Check sheet for the drawn part. Datum: minimum x, y, z corner. Units: mm. Round coordinates to 2 decimals unless told otherwise and drop trailing zeros. Write each loop counter-clockwise with the first axis right and the second up, starting at its lowest first coordinate (ties: lowest second). Pieces come first, ordered by that corner, then holes. Notation, with made-up numbers: (29, 5.25) - (73, 5.25) arc R16 cw to (73, 10.25) - close; hole circle Ø3 at (67, 68.5). An arc over 180 degrees is marked (long way). Write each question's results on one line, items separated by ' | '.
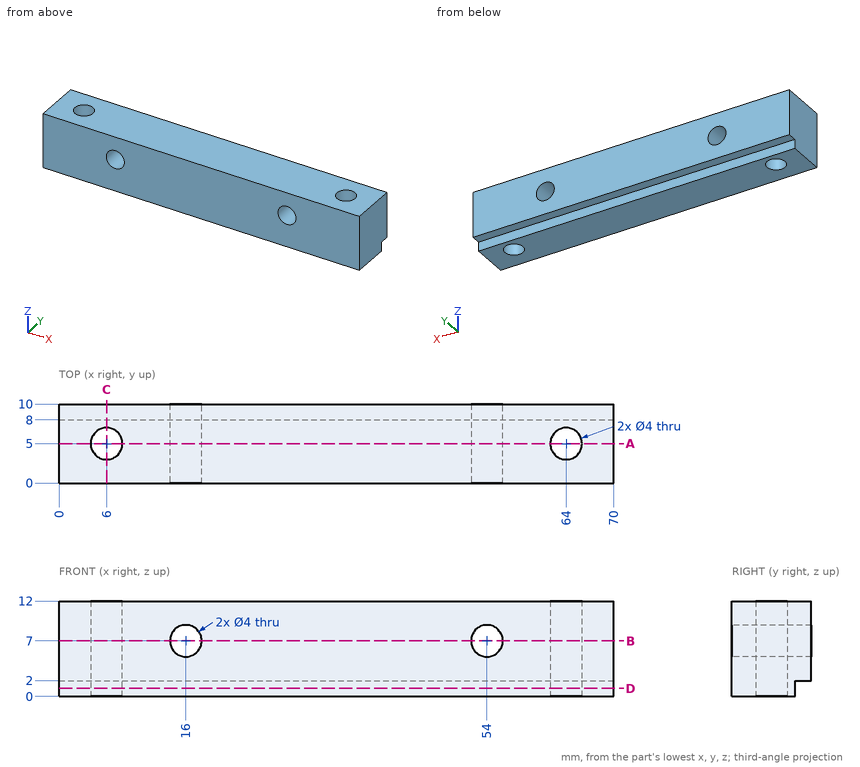
(1) Section check D-D (z = 1). Record the cut outline in (x, y), plus the area to 3 significant figures.
Answer:
outline: (0, 0) - (70, 0) - (70, 8) - (0, 8) - close; hole circle Ø4 at (6, 5); hole circle Ø4 at (64, 5) | area: 535 mm2
(2) Section check B-B (z = 7). Record the cut outline in (x, y), plus the area to 3 significant figures.
Answer:
outline: (0, 0) - (14, 0) - (14, 10) - (0, 10) - close; (18, 0) - (52, 0) - (52, 10) - (18, 10) - close; (56, 0) - (70, 0) - (70, 10) - (56, 10) - close; hole circle Ø4 at (6, 5); hole circle Ø4 at (64, 5) | area: 595 mm2
(3) Section check A-A (y = 5). Record the cut outline in (x, z), plus the area to 3 significant figures.
Answer:
outline: (0, 0) - (4, 0) - (4, 12) - (0, 12) - close; (8, 0) - (62, 0) - (62, 12) - (8, 12) - close; (66, 0) - (70, 0) - (70, 12) - (66, 12) - close; hole circle Ø4 at (16, 7); hole circle Ø4 at (54, 7) | area: 719 mm2
(4) Go/stop test with flat-tipped pins: pin 1 Ø2 at (x, z) = (25.5, 0.5) entering from +Y; pin 2 Ø1.6 at (x, y) = (18.5, 9) entering from -Z. Record where each tip stops, or that it passes through.
Answer:
pin 1: y = 8 | pin 2: z = 2
(5) Section check C-C (x = 6). Record the cut outline in (y, z).
Answer:
outline: (0, 0) - (3, 0) - (3, 12) - (0, 12) - close; (7, 0) - (8, 0) - (8, 2) - (10, 2) - (10, 12) - (7, 12) - close
(6) Thickness scan on L1, parallel to Z at x = 54, y = 2.25; L2, parallel to X at y = 6, z = 7.5; L3, parallel to Y at x = 6, z = 3.25. Record the ranges inside material, lowest first.
Answer:
L1: 0 to 5, 9 to 12 | L2: 0 to 4.27, 7.73 to 14.06, 17.94 to 52.06, 55.94 to 62.27, 65.73 to 70 | L3: 0 to 3, 7 to 10
